The drawing under review shows one solid part. Ordinate dimensions are in mm from its lowest x, y, z. A direction names the side the tool comes from. Give positions to 0.01 mm unless a question says otherwise; leave off trailing zeros. Loops run counter-clockwise (first coordinate to the right, second up) from the corner with the lowest first, then second, coordinate; pieces in that order, holes last. Notation, with made-up numbers: (46, 9) -> (76, 9) arc R34 ccw to (76, 43) -> close; hole circle Ø3 at (37.5, 6). An arc over 180 degrees is marked (long way). Answer in a Markdown table with one row per item. Add a question column.
(1) Consider section A-A on x = 15. Write out the cut boundary in (y, z), then the cut area to 3 significant figures.
(2) For line 1 (Y direction, x = 14.75, z = 62); line 2 (Z direction, x = 9.5, y = 28.75); line 3 (X direction, y = 20, z = 107.5), list the stretches that pass through material, from the lowest coordinate up.
(3) Consider section C-C on z = 31. Write out the cut boundary in (x, y).
(4) For the marked faces 1, 2 and 3, list the 3-axis set-ups (+Z, -Z, +X, -X, +Y, -Y) from which the entire face can be reached by the end or side of a thin tool; tool diameter is ignored.
(5) For pin 1 (1 mm diameter, centred on x = 22.5, z = 50, fed in from -Y); pin 2 (8 mm diameter, centred on x = 19.5, z = 31.5, fed in from -Y); pin 3 (12 mm diameter, centred on x = 6.5, z = 80.5, fed in from -Y), all flat-tipped, find the tip position at first contact; note any pin that passes through.
(6) Consider section D-D on x = 24. Write out the cut boundary in (y, z), then the cut area to 3 significant figures.
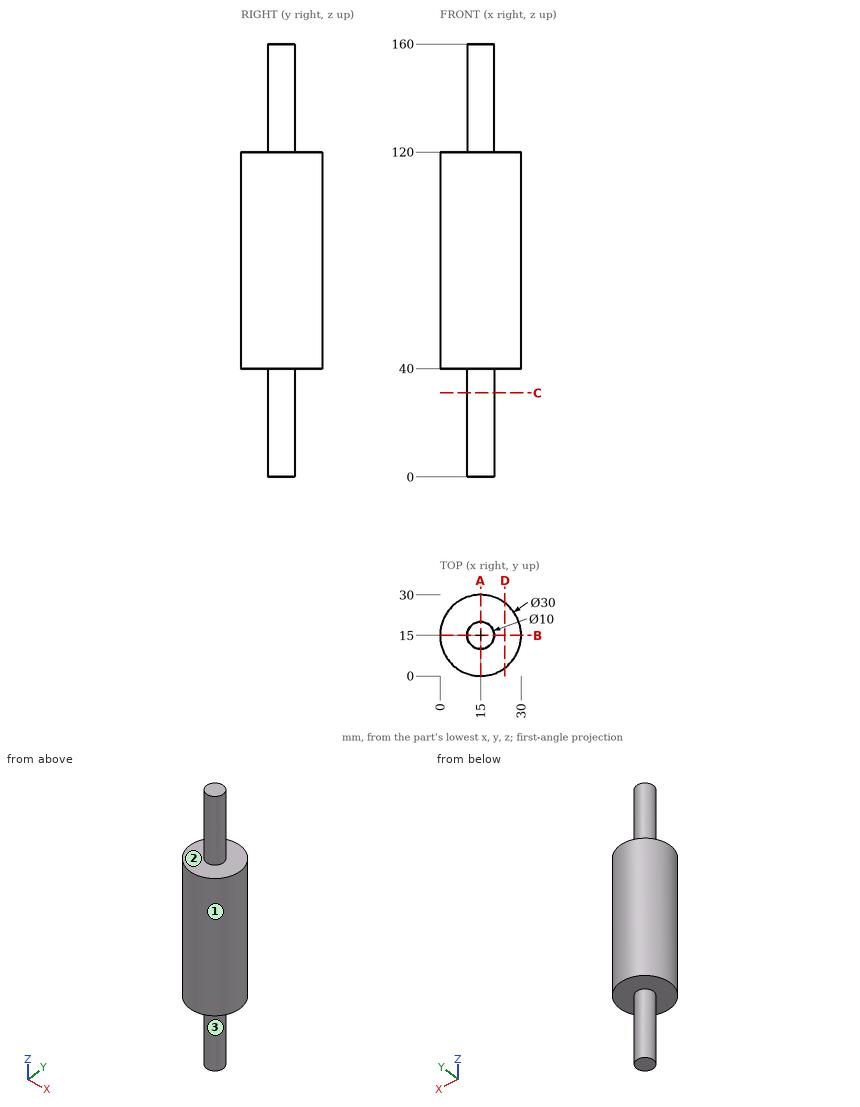
Values follow:
| question | item | result |
|---|---|---|
| 1 | outline | (0, 40) -> (10, 40) -> (10, 0) -> (20, 0) -> (20, 40) -> (30, 40) -> (30, 120) -> (20, 120) -> (20, 160) -> (10, 160) -> (10, 120) -> (0, 120) -> close |
| 1 | area | 3,200 mm2 |
| 2 | line 1 | 0 to 30 |
| 2 | line 2 | 40 to 120 |
| 2 | line 3 | 0.86 to 29.14 |
| 3 | outline | circle Ø10 at (15, 15) |
| 4 | face 1 | +Z, -Z |
| 4 | face 2 | +Z |
| 4 | face 3 | -Z |
| 5 | pin 1 | y = 1.73 |
| 5 | pin 2 | y = 10.03 |
| 5 | pin 3 | y = 0.21 |
| 6 | outline | (3, 40) -> (27, 40) -> (27, 120) -> (3, 120) -> close |
| 6 | area | 1,920 mm2 |
